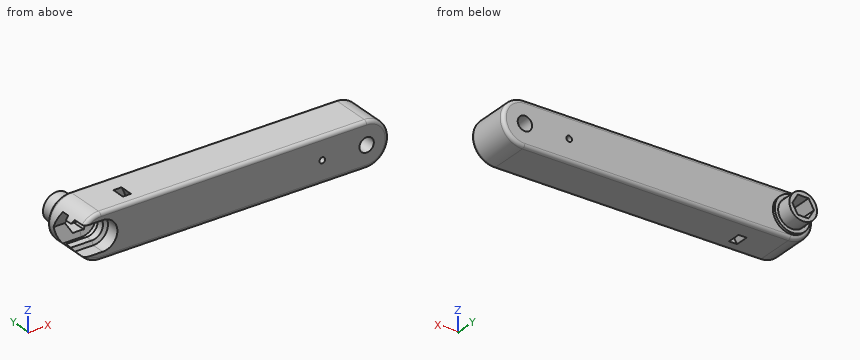
from build123d import *

# Parameters (mm, degrees)
SALIENTE_EXTRUIR1_DEPTH    = 25
CROQUIS5_R                 = 4.05
CROQUIS5_R_2               = 1.6
CORTAR_EXTRUIR1_DEPTH      = 51.5
REDONDEO2_R                = 2
CORTAR_EXTRUIR2_REACH      = 168.696
CORTAR_EXTRUIR4_DEPTH      = 1
CORTAR_EXTRUIR4_DEPTH_BACK = 167.695830887
CROQUIS13_W                = 3.831890827
CROQUIS13_H                = 7.53605196


with BuildPart() as part:
    # Croquis2 → Saliente-Extruir1 (new body)
    with BuildSketch(Plane(origin=(0, 0, 0), x_dir=(1, 0, 0), z_dir=(0, 1, 0))):
        with BuildLine():
            Line((0, -12.5), (150, -12.5))
            ThreePointArc((150, -12.5), (162.5, 0), (150, 12.5))
            Line((150, 12.5), (0, 12.5))
            ThreePointArc((0, 12.5), (-12.5, 0), (0, -12.5))
        make_face()
    extrude(amount=SALIENTE_EXTRUIR1_DEPTH)

    # Croquis5 → Cortar-Extruir1 (cut)
    with BuildSketch(Plane(origin=(0, 25, 0), x_dir=(1, 0, 0), z_dir=(0, 1, 0))):
        with Locations(Location((150, 0, 0), (0, 0, 270))):
            Circle(CROQUIS5_R)
        with Locations(Location((125, 0, 0), (0, 0, 270))):
            Circle(CROQUIS5_R_2)
    extrude(amount=-CORTAR_EXTRUIR1_DEPTH, mode=Mode.SUBTRACT)

    # Croquis9 → Revolución2 (revolve)
    with BuildSketch(Plane.XY, mode=Mode.PRIVATE) as revoluci_n2_sk:
        Polygon((0, 25), (0, 35), (7.8, 35), (7.8, 26.5), (7.8, 26.1), (8.2, 26.1), (8.2, 26.5), (10, 26.5), (10, 25), align=None)
    revolve(revoluci_n2_sk.sketch.rotate(Axis((0, 25, 0), (0, 1, 0)), 90), axis=Axis((0, 25, 0), (0, 1, 0)))

    # Croquis1 → Cortar-Revolución1 (revolve, cut)
    with BuildSketch(Plane.XY, mode=Mode.PRIVATE) as cortar_revoluci_n1_sk:
        Polygon((9.3, 17), (1, 20), (1, 0), (9.3, 0), (9.3, 7.5), (7.3, 8.654700538), (7.3, 12.7), (9.3, 12.7), align=None)
    revolve(cortar_revoluci_n1_sk.sketch.rotate(Axis((1, 20, 0), (0, -1, 0)), 180), axis=Axis((1, 20, 0), (0, -1, 0)), mode=Mode.SUBTRACT)

    # Redondeo2
    redondeo2_edges = [part.edges().sort_by_distance(p)[0] for p in [
        (162.5, 25, 0),
        (75, 25, -12.5),
        (-12.5, 25, 0),
        (75, 0, -12.5),
        (162.5, 0, 0),
        (75, 0, 12.5),
        (-12.5, 0, 0),
        (75, 25, 12.5),
    ]]
    fillet(redondeo2_edges, radius=REDONDEO2_R)

    # Cortar-Extruir2: up to this cone (the profile starts outside it)
    cortar_extruir2_end = Plane(origin=(1, 35, 0), z_dir=(0, -1, 0)).offset(15.000001) * Cone(2.767e-06, 426.608933333, 154.195999, align=(Align.CENTER, Align.CENTER, Align.MIN), mode=Mode.PRIVATE)
    # Croquis10 → Cortar-Extruir2 (cut, up to the surface)
    with BuildSketch(Plane(origin=(0, 35, 0), x_dir=(1, 0, 0), z_dir=(0, 1, 0)), mode=Mode.PRIVATE) as cortar_extruir2_sk1:
        Polygon((6.119912853, 0), (3.059956427, 5.3), (-3.059956427, 5.3), (-6.119912853, 0), (-3.059956427, -5.3), (3.059956427, -5.3), align=None)
    cortar_extruir2_tool1 = extrude(cortar_extruir2_sk1.sketch, amount=-CORTAR_EXTRUIR2_REACH, mode=Mode.PRIVATE) - cortar_extruir2_end
    add(cortar_extruir2_tool1.solids().sort_by_distance((0, 35, 0))[0], mode=Mode.SUBTRACT)

    # Croquis12 → Cortar-Extruir4 (cut, two sides: drawn at the far end of the back side and taken through both)
    with BuildSketch(Plane(origin=(0, 0, 0), x_dir=(0, 0, -1), z_dir=(1, 0, 0)).offset(-CORTAR_EXTRUIR4_DEPTH_BACK)):
        Polygon((8.3, 7.5), (6.3, 8.654700538), (6.3, 12.7), (8.3, 12.7), (8.3, 17), (0, 20), (-8.3, 17), (-8.3, 12.7), (-6.3, 12.7), (-6.3, 8.654700538), (-8.3, 7.5), (-8.3, 0), (8.3, 0), align=None)
    extrude(amount=CORTAR_EXTRUIR4_DEPTH + CORTAR_EXTRUIR4_DEPTH_BACK, mode=Mode.SUBTRACT)

    # Croquis13 → Cortar-Revolución2 (revolve, cut)
    with BuildSketch(Plane.XY):
        with Locations((23.136343839, 10.430899618)):
            Rectangle(CROQUIS13_W, CROQUIS13_H)
    revolve(axis=Axis((0, 0, 0), (0, 1, 0)), mode=Mode.SUBTRACT)


solid = part.part
For this review, take the finished solid that the model builds, in its own axes (mm). Round coordinates to 2 decimals unless told otherwise and drop trailing zeros. Order: outer loops, then holes, each group sorted by start corner. A loop starts at its lowest first (then second) coordinate and runs counter-clockwise, first axis right, second up. Notation, with made-up numbers: M -11,36 L 24,36 A28 ccw 24,60 Z; hole C 52.25,58 d4. An arc over 180 degrees is marked long. Write each question's results on one line, items separated by ' | '. Start each with the question number.
1. Add section B-B (y = 28.5). State the section outline as (x, z) points.
2. Add section D-D (x = 148). State the section outline as (y, z) points, then the cut area to 3 significant figures.
3. Add section A-A (x = 125). State the section outline as (y, z) points.
4. Clearance check with flat-ended pins moving along their axes: pin 1 Ø4 at (x, y) = (-5.5, 3) entering from +Z; pin 2 Ø1.5 at (y, z) = (15, -10) entering from -X; pin 3 Ø12 at (y, z) = (20.5, -6.5) entering from +X; pin 4 Ø2.5 at (x, z) = (125, 0) entering from -Y. State where each tip first meets the part, or that it passes through.
5. Add section C-C (x = 44.5). State the section outline as (y, z) points, then the cut area to 3 significant figures.
6. To check wall thickness, follow L1, parallel to X at y = 6.25, z = 0; L2, parallel to X at y = 19.25, z = 0; L3, parallel to X at y = 26.25, z = 0. State the ranges of each line that lie inside material, in increasing order. Write a range as [from, to].
Output values:
1) outline: C 0,0 d15.6; hole M -6.12,0 L -3.06,-5.3 L 3.06,-5.3 L 6.12,0 L 3.06,5.3 L -3.06,5.3 Z
2) outline: M 0,-10.5 A2 ccw 2,-12.5 L 23,-12.5 A2 ccw 25,-10.5 L 25,-3.52 L 0,-3.52 Z; M 0,3.52 L 25,3.52 L 25,10.5 A2 ccw 23,12.5 L 2,12.5 A2 ccw 0,10.5 Z | area: 445 mm^2
3) outline: M 0,-10.5 A2 ccw 2,-12.5 L 23,-12.5 A2 ccw 25,-10.5 L 25,-1.6 L 0,-1.6 Z; M 0,1.6 L 25,1.6 L 25,10.5 A2 ccw 23,12.5 L 2,12.5 A2 ccw 0,10.5 Z
4) pin 1: z = 12 | pin 2: x = -8.41 | pin 3: x = 162.49 | pin 4: through
5) outline: M 0,-10.5 A2 ccw 2,-12.5 L 23,-12.5 A2 ccw 25,-10.5 L 25,10.5 A2 ccw 23,12.5 L 2,12.5 A2 ccw 0,10.5 Z | area: 622 mm^2
6) L1: [9.3, 123.4], [126.6, 145.95], [154.05, 162.5] | L2: [6.12, 123.4], [126.6, 145.95], [154.05, 162.5] | L3: [-10, -8.2], [-7.8, -6.12], [6.12, 7.8], [8.2, 10]
